Check sheet for the modelled part. Datum: model origin and axes. Units: mm. Face numbers are marked on the shaded views. A direction names the side the tool comes from. Give positions to 0.01 mm unless a question says otherwise; leave off trailing zeros. Write each loop counter-clockwise with the first axis right and the second up, starting at its lowest first coordinate (ties: lowest second). Pieces come first, ordered by that corner, then holes. Notation, with made-up numbers: M 10.5,22 L 20.5,22 A10 cw 20.5,36 Z; hole C 13,7.5 d3. An arc over 180 degrees is marked long. Write item = value, one per line. Start each with the question number.
1) Set-up check for the marked faces 1, 2, 3 and 4: record each of +Z, -Z, +X, -X, +Y, -Y from which the full face is reachable in a straight line by a thin tool's end or side.
2) Sectioned sample at B-B, the plane y = 40. Record the cut outline in (x, z), then the cut area to 3 significant figures.
3) Scan lines: L1, parallel to Y at x = 0, z = 27.75; L2, parallel to Y at x = 24.5, z = 15; L3, parallel to X at y = 3, z = 12. Record each from-to range of solid material in increasing order.
4) Sectioned sample at C-C, the plane z = 5.5. Record the cut outline in (x, y).
5) Sectioned sample at D-D, the plane y = 9. Record the cut outline in (x, z) (3 decimals), then the cut area to 3 significant figures.
6) Gauge pin test, flat ends, axial feed: pin 1 (3.5 mm diameter, centred on y = 8, z = 18, fed in from +X); pin 2 (8.5 mm diameter, centred on x = 0, y = 38.53, fed in from -Z); pin 3 (8 mm diameter, centred on y = 21, z = 25.5, fed in from -X); pin 4 (4 mm diameter, centred on x = 38.53, y = 0, fed in from +Z). Record the tip position at first contact, or that the pin passes through.
7) Sectioned sample at A-A, the plane z = 12.75. Record the cut outline in (x, y).
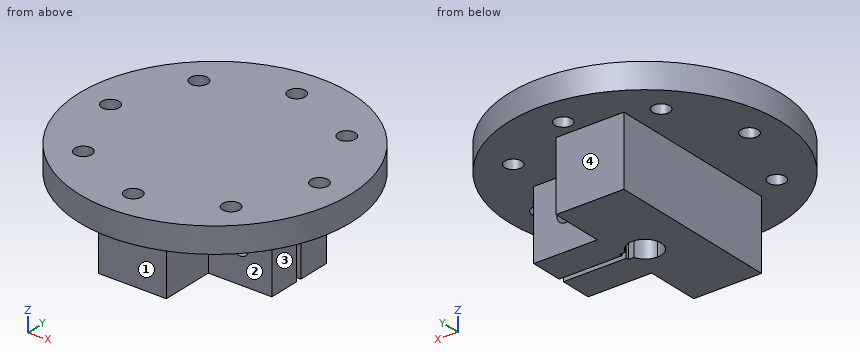
from build123d import *

# Parameters (mm, degrees)
SKETCH_1_W           = 30
SKETCH_1_H           = 14.828427124
EXTRUDE_2_DEPTH      = 25.5
CUT_EXTRUDE_9_DEPTH  = 46
CUT_EXTRUDE_10_DEPTH = 30
CUT_EXTRUDE_11_DEPTH = 31
CUT_EXTRUDE_12_DEPTH = 40
SKETCH_1_15_R        = 6
CUT_EXTRUDE_13_DEPTH = 46
CUT_EXTRUDE_17_DEPTH = 97
CUT_EXTRUDE_18_DEPTH = 285
SKETCH_12_R          = 50
EXTRUDE_7_DEPTH      = 9.398
SKETCH_16_W          = 11
SKETCH_16_H          = 2
CUT_EXTRUDE_25_DEPTH = 25.5
SKETCH_12_5_R        = 3.175
CUT_EXTRUDE_27_DEPTH = 63
SKETCH_20_W          = 10
SKETCH_20_H          = 20
SKETCH_20_H_2        = 19.641492006
SKETCH_20_W_2        = 10.171572876
SKETCH_20_H_3        = 14.828427124
EXTRUDE_9_DEPTH      = 26
SKETCH_20_8_W        = 10
SKETCH_20_8_H        = 2
EXTRUDE_10_DEPTH     = 26
SKETCH_21_R          = 3.175
CUT_EXTRUDE_28_DEPTH = 54
SKETCH_22_W          = 23.435889716
SKETCH_22_H          = 10
CUT_EXTRUDE_31_DEPTH = 25.5
SKETCH_1_26_W        = 0.7
SKETCH_1_26_H        = 1
CUT_EXTRUDE_32_DEPTH = 25.5


with BuildPart() as part:
    # Sketch 1 → Extrude 2 (new body)
    with BuildSketch(Plane.XY):
        with Locations((7.585786438, 0)):
            Rectangle(SKETCH_1_W, SKETCH_1_H)
    extrude(amount=EXTRUDE_2_DEPTH)

    # Sketch 1_11 → Cut-Extrude 9 (cut)
    with BuildSketch(Plane.XY):
        with BuildLine():
            Line((0, -2), (0, 0))
            Line((0, 0), (-6, 0))
            ThreePointArc((-6, 0), (-4.242640687, -4.242640687), (0, -6))
            ThreePointArc((0, -6), (3.464101615, -4.898979486), (5.656854249, -2))
            Line((5.656854249, -2), (0, -2))
        make_face()
    extrude(amount=CUT_EXTRUDE_9_DEPTH, mode=Mode.SUBTRACT)

    # Sketch 1_12 → Cut-Extrude 10 (cut)
    with BuildSketch(Plane.XY):
        with BuildLine():
            Line((-6, 0), (0, 0))
            Line((0, 0), (0, 2))
            Line((0, 2), (0, 6))
            ThreePointArc((0, 6), (-4.242640687, 4.242640687), (-6, 0))
        make_face()
    extrude(amount=CUT_EXTRUDE_10_DEPTH, mode=Mode.SUBTRACT)

    # Sketch 1_13 → Cut-Extrude 11 (cut)
    with BuildSketch(Plane.XY):
        with BuildLine():
            Line((0, 2), (0, 0))
            Line((0, 0), (6, 0))
            ThreePointArc((6, 0), (5.913591358, 1.014611872), (5.656854249, 2))
            Line((5.656854249, 2), (0, 2))
        make_face()
    extrude(amount=CUT_EXTRUDE_11_DEPTH, mode=Mode.SUBTRACT)

    # Sketch 1_14 → Cut-Extrude 12 (cut)
    with BuildSketch(Plane.XY):
        with BuildLine():
            Line((6, 0), (0, 0))
            Line((0, 0), (0, -2))
            Line((0, -2), (5.656854249, -2))
            ThreePointArc((5.656854249, -2), (5.913591358, -1.014611872), (6, 0))
        make_face()
    extrude(amount=CUT_EXTRUDE_12_DEPTH, mode=Mode.SUBTRACT)

    # Sketch 1_15 → Cut-Extrude 13 (cut)
    with BuildSketch(Plane.XY):
        Circle(SKETCH_1_15_R)
    extrude(amount=CUT_EXTRUDE_13_DEPTH, mode=Mode.SUBTRACT)

    # Sketch 1_19 → Cut-Extrude 17 (cut)
    with BuildSketch(Plane.XY):
        with BuildLine():
            ThreePointArc((5.656854249, 2), (5.913591358, 1.014611872), (6, 0))
            Line((6, 0), (6, 2))
            Line((6, 2), (5.656854249, 2))
        make_face()
        Polygon((6, 2), (6, 0), (7, 0), (7, 1), (7, 2), align=None)
        Polygon((7, 0), (6, 0), (6, -2), (7, -2), (7, -1), align=None)
        with BuildLine():
            Line((6, -2), (6, 0))
            ThreePointArc((6, 0), (5.913591358, -1.014611872), (5.656854249, -2))
            Line((5.656854249, -2), (6, -2))
        make_face()
    extrude(amount=CUT_EXTRUDE_17_DEPTH, mode=Mode.SUBTRACT)

    # Sketch 1_20 → Cut-Extrude 18 (cut)
    with BuildSketch(Plane.XY):
        with BuildLine():
            ThreePointArc((7.414213562, 7.414213562), (9.005239827, 5.370919954), (10.046946078, 3))
            Line((10.046946078, 3), (18, 3))
            Line((18, 3), (20.850103278, 3))
            Line((20.850103278, 3), (20.850103278, 1))
            Line((20.850103278, 1), (18, 1))
            Line((18, 1), (18, -1))
            Line((18, -1), (20.850103278, -1))
            Line((20.850103278, -1), (20.850103278, -3))
            Line((20.850103278, -3), (18, -3))
            Line((18, -3), (10.046946078, -3))
            ThreePointArc((10.046946078, -3), (9.005239827, -5.370919954), (7.414213562, -7.414213562))
            Line((7.414213562, -7.414213562), (22.585786438, -7.414213562))
            Line((22.585786438, -7.414213562), (22.585786438, 7.414213562))
            Line((22.585786438, 7.414213562), (7.414213562, 7.414213562))
        make_face()
    extrude(amount=CUT_EXTRUDE_18_DEPTH, mode=Mode.SUBTRACT)

    # Sketch 12 → Extrude 7 (add)
    with BuildSketch(Plane.XY.offset(25.5)):
        Circle(SKETCH_12_R)
    extrude(amount=EXTRUDE_7_DEPTH)

    # Sketch 16 → Cut-Extrude 25 (cut)
    with BuildSketch(Plane(origin=(0, 0, 0), x_dir=(-1, 0, 0), z_dir=(0, 0, -1))):
        with Locations((-12.5, 0)):
            Rectangle(SKETCH_16_W, SKETCH_16_H)
    extrude(amount=-CUT_EXTRUDE_25_DEPTH, mode=Mode.SUBTRACT)

    # Sketch 12_5 → Cut-Extrude 27 (cut)
    with BuildSketch(Plane.XY.offset(25.5)):
        with Locations((27.24506403, 27.24506403)):
            Circle(SKETCH_12_5_R)
        with Locations((-27.24506403, 27.24506403)):
            Circle(SKETCH_12_5_R)
        with Locations((-38.530339059, 0)):
            Circle(SKETCH_12_5_R)
        with Locations((-27.24506403, -27.24506403)):
            Circle(SKETCH_12_5_R)
        with Locations((0, -38.530339059)):
            Circle(SKETCH_12_5_R)
        with Locations((27.24506403, -27.24506403)):
            Circle(SKETCH_12_5_R)
        with Locations((38.530339059, 0)):
            Circle(SKETCH_12_5_R)
        with Locations((0, 38.530339059)):
            Circle(SKETCH_12_5_R)
    extrude(amount=CUT_EXTRUDE_27_DEPTH, mode=Mode.SUBTRACT)

    # Sketch 20 → Extrude 9 (add)
    with BuildSketch(Plane(origin=(0, 0, 0), x_dir=(-1, 0, 0), z_dir=(0, 0, -1))):
        Polygon((-7.414213562, 23), (-7.414213562, 7.414213562), (7.414213562, 7.414213562), (17.585786438, 7.414213562), (17.585786438, 32.414213562), (-7.414213562, 32.414213562), align=None)
        with BuildLine():
            ThreePointArc((-10.046946078, 3), (-9.005239827, 5.370919954), (-7.414213562, 7.414213562))
            Line((-7.414213562, 7.414213562), (-7.414213562, 23))
            Line((-7.414213562, 23), (-20.850103278, 23))
            Line((-20.850103278, 23), (-20.850103278, 3))
            Line((-20.850103278, 3), (-10.046946078, 3))
        make_face()
        with Locations((-25.850103278, 13)):
            Rectangle(SKETCH_20_W, SKETCH_20_H)
        with Locations((-25.850103278, -12.820746003)):
            Rectangle(SKETCH_20_W, SKETCH_20_H_2)
        with BuildLine():
            Line((-7.414213562, -22.641492006), (-7.414213562, -7.414213562))
            ThreePointArc((-7.414213562, -7.414213562), (-9.005239827, -5.370919954), (-10.046946078, -3))
            Line((-10.046946078, -3), (-20.850103278, -3))
            Line((-20.850103278, -3), (-20.850103278, -22.641492006))
            Line((-20.850103278, -22.641492006), (-7.414213562, -22.641492006))
        make_face()
        Polygon((17.585786438, -7.414213562), (7.414213562, -7.414213562), (-7.414213562, -7.414213562), (-7.414213562, -22.641492006), (-7.414213562, -32.414213562), (17.585786438, -32.414213562), align=None)
        with Locations((12.5, 0)):
            Rectangle(SKETCH_20_W_2, SKETCH_20_H_3)
        with BuildLine():
            ThreePointArc((-10.046946078, -3), (-9.005239827, -5.370919954), (-7.414213562, -7.414213562))
            Line((-7.414213562, -7.414213562), (-7.414213562, -3))
            Line((-7.414213562, -3), (-10.046946078, -3))
        make_face()
        with BuildLine():
            Line((-7.414213562, 3), (-7.414213562, 7.414213562))
            ThreePointArc((-7.414213562, 7.414213562), (-9.005239827, 5.370919954), (-10.046946078, 3))
            Line((-10.046946078, 3), (-7.414213562, 3))
        make_face()
    extrude(amount=-EXTRUDE_9_DEPTH)

    # Sketch 20_8 → Extrude 10 (add)
    with BuildSketch(Plane(origin=(0, 0, 0), x_dir=(-1, 0, 0), z_dir=(0, 0, -1))):
        with Locations((-25.850103278, 2)):
            Rectangle(SKETCH_20_8_W, SKETCH_20_8_H)
        with Locations((-25.850103278, -2)):
            Rectangle(SKETCH_20_8_W, SKETCH_20_8_H)
    extrude(amount=-EXTRUDE_10_DEPTH)

    # Sketch 21 → Cut-Extrude 28 (cut)
    with BuildSketch(Plane.XZ.offset(22.641492006)):
        with Locations((19.13215842, 12.75)):
            Circle(SKETCH_21_R)
    extrude(amount=-CUT_EXTRUDE_28_DEPTH, mode=Mode.SUBTRACT)

    # Sketch 22 → Cut-Extrude 31 (cut)
    with BuildSketch(Plane(origin=(0, 0, 0), x_dir=(-1, 0, 0), z_dir=(0, 0, -1))):
        with Locations((-19.13215842, -17.641492006)):
            Rectangle(SKETCH_22_W, SKETCH_22_H)
        with Locations((-19.13215842, 18)):
            Rectangle(SKETCH_22_W, SKETCH_22_H)
    extrude(amount=-CUT_EXTRUDE_31_DEPTH, mode=Mode.SUBTRACT)

    # Sketch 1_26 → Cut-Extrude 32 (cut)
    with BuildSketch(Plane.XY):
        with Locations((7.35, 1.5)):
            Rectangle(SKETCH_1_26_W, SKETCH_1_26_H)
        with Locations((7.35, -1.5)):
            Rectangle(SKETCH_1_26_W, SKETCH_1_26_H)
    extrude(amount=CUT_EXTRUDE_32_DEPTH, mode=Mode.SUBTRACT)


solid = part.part
Data:
q1.face_1 = -Z, +X, -X, -Y
q1.face_2 = -Z, +X, -Y
q1.face_3 = -Z, +X, +Y, -Y
q1.face_4 = -Z, +X, -X, +Y
q2.outline = M -30,25.5 L -2.81,25.5 L -2.81,34.9 L -30,34.9 Z; M 2.81,25.5 L 30,25.5 L 30,34.9 L 2.81,34.9 Z
q2.area = 511 mm2
q3.L1 = -50 to -41.71, -35.36 to 35.36, 41.71 to 50
q3.L2 = -12.64 to -1, 1 to 13
q3.L3 = -17.59 to -5.2, 5.2 to 16.05, 22.22 to 30.85
q4.outline = M -17.59,-32.41 L 7.41,-32.41 L 7.41,-12.64 L 30.85,-12.64 L 30.85,-1 L 7.7,-1 L 7.7,-2 L 5.66,-2 A6 cw long 5.66,2 L 7.7,2 L 7.7,1 L 30.85,1 L 30.85,13 L 7.41,13 L 7.41,32.41 L -17.59,32.41 Z
q5.outline = M -49.183,25.5 L -17.586,25.5 L -17.586,0 L 30.85,0 L 30.85,25.5 L 49.183,25.5 L 49.183,34.898 L -49.183,34.898 Z; hole C 19.132,12.75 d6.35
q5.area = 2,130 mm2
q6.pin_1 = 30.85
q6.pin_2 = 25.5
q6.pin_3 = -47.02
q6.pin_4 = through
q7.outline = M -17.59,-32.41 L 7.41,-32.41 L 7.41,-12.64 L 15.96,-12.64 L 15.96,-1 L 7.7,-1 L 7.7,-2 L 5.66,-2 A6 cw long 5.66,2 L 7.7,2 L 7.7,1 L 15.96,1 L 15.96,13 L 7.41,13 L 7.41,32.41 L -17.59,32.41 Z; M 22.31,-12.64 L 30.85,-12.64 L 30.85,-1 L 22.31,-1 Z; M 22.31,1 L 30.85,1 L 30.85,13 L 22.31,13 Z
